from build123d import *

# Parameters (mm, degrees)
SKETCH_2_W          = 210
SKETCH_2_H          = 67
SKETCH_2_W_2        = 50
SKETCH_2_H_2        = 63
EXTRUDE_1_DEPTH     = 143
SKETCH_3_W          = 210
SKETCH_3_H          = 67
EXTRUDE_2_DEPTH     = 2
CUT_EXTRUDE_1_DEPTH = 5
SKETCH_5_W          = 210
SKETCH_5_H          = 145
CUT_EXTRUDE_2_DEPTH = 3
SKETCH_6_R          = 3.5
EXTRUDE_3_DEPTH     = 5
SKETCH_7_W          = 39
SKETCH_7_H          = 22
EXTRUDE_4_DEPTH     = 47
SKETCH_8_R          = 2.75
EXTRUDE_5_DEPTH     = 15
CUT_EXTRUDE_3_DEPTH = 288.697758073
FILLET_1_R          = 10
FILLET_2_R          = 4
EXTRUDE_6_DEPTH     = 5
FILLET_3_R          = 5
FILLET_4_R          = 2
SKETCH_11_W         = 210
SKETCH_11_H         = 49
CUT_EXTRUDE_4_DEPTH = 5
FILLET_5_R          = 5


# Some blends are built 0.0001 mm under size
with BuildPart() as part:
    # Эскиз2 → Бобышка-Вытянуть1 (new body)
    with BuildSketch(Plane.XY):
        with Locations((100, 28.5)):
            Rectangle(SKETCH_2_W, SKETCH_2_H)
        with Locations((22, 28.5)):
            Rectangle(SKETCH_2_W_2, SKETCH_2_H_2, mode=Mode.SUBTRACT)
        with Locations((74, 28.5)):
            Rectangle(SKETCH_2_W_2, SKETCH_2_H_2, mode=Mode.SUBTRACT)
        with Locations((126, 28.5)):
            Rectangle(SKETCH_2_W_2, SKETCH_2_H_2, mode=Mode.SUBTRACT)
        with Locations((178, 28.5)):
            Rectangle(SKETCH_2_W_2, SKETCH_2_H_2, mode=Mode.SUBTRACT)
    extrude(amount=EXTRUDE_1_DEPTH)

    # Эскиз3 → Бобышка-Вытянуть2 (add)
    with BuildSketch(Plane.XY.offset(143)):
        with Locations((100, 28.5)):
            Rectangle(SKETCH_3_W, SKETCH_3_H)
    extrude(amount=EXTRUDE_2_DEPTH)

    # Эскиз4 → Вырез-Вытянуть1 (cut)
    with BuildSketch(Plane.XZ.offset(5)):
        with BuildLine():
            Line((85.828427125, 143), (114.171572875, 143))
            ThreePointArc((114.171572875, 143), (115.319623172, 143.228361402), (116.292893219, 143.878679656))
            Line((116.292893219, 143.878679656), (118.414213562, 146))
            Line((118.414213562, 146), (81.585786438, 146))
            Line((81.585786438, 146), (83.707106781, 143.878679656))
            ThreePointArc((83.707106781, 143.878679656), (84.680376828, 143.228361402), (85.828427125, 143))
        make_face()
    extrude(amount=-CUT_EXTRUDE_1_DEPTH, mode=Mode.SUBTRACT)

    # Эскиз5 → Вырез-Вытянуть2 (cut)
    with BuildSketch(Plane(origin=(0, 62, 0), x_dir=(1, 0, 0), z_dir=(0, 1, 0))):
        with Locations((100, -72.5)):
            Rectangle(SKETCH_5_W, SKETCH_5_H)
    extrude(amount=-CUT_EXTRUDE_2_DEPTH, mode=Mode.SUBTRACT)

    # Эскиз6 → Бобышка-Вытянуть3 (add)
    # profile 1 of 4: a face of its own
    with BuildSketch(Plane.XZ.offset(5)):
        with BuildLine():
            Line((205, 22), (205, 39))
            Line((205, 39), (209, 39))
            ThreePointArc((209, 39), (217.5, 30.5), (209, 22))
            Line((209, 22), (205, 22))
        make_face()
        with Locations(Location((209, 30.5, 0), (0, 0, 270))):
            Circle(SKETCH_6_R, mode=Mode.SUBTRACT)
    # profile 2 of 4: a face of its own
    with BuildSketch(Plane.XZ.offset(5)):
        with BuildLine():
            Line((209, 47), (205, 47))
            Line((205, 47), (205, 64))
            Line((205, 64), (209, 64))
            ThreePointArc((209, 64), (217.5, 55.5), (209, 47))
        make_face()
        with Locations(Location((209, 55.5, 0), (0, 0, 270))):
            Circle(SKETCH_6_R, mode=Mode.SUBTRACT)
    # profile 3 of 4: a face of its own
    with BuildSketch(Plane.XZ.offset(5)):
        with BuildLine():
            Line((-5, 47), (-5, 64))
            Line((-5, 64), (-9, 64))
            ThreePointArc((-9, 64), (-17.5, 55.5), (-9, 47))
            Line((-9, 47), (-5, 47))
        make_face()
        with Locations(Location((-9, 55.5, 0), (0, 0, 90))):
            Circle(SKETCH_6_R, mode=Mode.SUBTRACT)
    # profile 4 of 4: a face of its own
    with BuildSketch(Plane.XZ.offset(5)):
        with BuildLine():
            Line((-9, 39), (-5, 39))
            Line((-5, 39), (-5, 22))
            Line((-5, 22), (-9, 22))
            ThreePointArc((-9, 22), (-17.5, 30.5), (-9, 39))
        make_face()
        with Locations(Location((-9, 30.5, 0), (0, 0, 90))):
            Circle(SKETCH_6_R, mode=Mode.SUBTRACT)
    extrude(amount=-EXTRUDE_3_DEPTH)

    # Эскиз7 → Бобышка-Вытянуть4 (add)
    with BuildSketch(Plane.XZ.offset(5)):
        with Locations((224.5, 11)):
            Rectangle(SKETCH_7_W, SKETCH_7_H)
    extrude(amount=-EXTRUDE_4_DEPTH)

    # Эскиз8 → Бобышка-Вытянуть5 (add)
    with BuildSketch(Plane.XZ.offset(-42)):
        with BuildLine():
            Line((239, 23), (217, 23))
            ThreePointArc((217, 23), (213.464466094, 21.535533906), (212, 18))
            Line((212, 18), (212, -29.15))
            ThreePointArc((212, -29.15), (213.464466094, -32.685533906), (217, -34.15))
            Line((217, -34.15), (239, -34.15))
            ThreePointArc((239, -34.15), (242.535533906, -32.685533906), (244, -29.15))
            Line((244, -29.15), (244, 18))
            ThreePointArc((244, 18), (242.535533906, 21.535533906), (239, 23))
        make_face()
        with Locations(Location((238.75, -5.575, 0), (0, 0, 270))):
            Circle(SKETCH_8_R, mode=Mode.SUBTRACT)
        with Locations(Location((217.25, -5.575, 0), (0, 0, 270))):
            Circle(SKETCH_8_R, mode=Mode.SUBTRACT)
    extrude(amount=EXTRUDE_5_DEPTH)

    # Эскиз9 → Вырез-Вытянуть3 (cut, through all)
    with BuildSketch(Plane(origin=(0, 42, 0), x_dir=(1, 0, 0), z_dir=(0, 1, 0))):
        with BuildLine():
            Line((239, -23), (235.274216073, -23))
            Line((235.274216073, -23), (246.59675483, -31.709945179))
            Line((246.59675483, -31.709945179), (255.697113083, -21.551405734))
            Line((255.697113083, -21.551405734), (244, -13.403410553))
            Line((244, -13.403410553), (244, -18))
            ThreePointArc((244, -18), (242.535533906, -21.535533906), (239, -23))
        make_face()
    extrude(amount=-CUT_EXTRUDE_3_DEPTH, mode=Mode.SUBTRACT)

    # Скругление1
    # the kernel refuses this fillet: 10 mm, written as the material it adds along each edge
    with BuildSketch(Plane(origin=(212, 66.874685928, 0), x_dir=(0, 0, -1), z_dir=(0, -1, 0))) as fillet_1_piece_1_section:
        with BuildLine():
            CenterArc((9.949874371, -10), FILLET_1_R, 90, 84.260829523)
            Line((0, -9), (0, 0))
            Line((0, 0), (9.949874371, 0))
        make_face()
    fillet_1_piece_1 = extrude(amount=39.874685928, mode=Mode.PRIVATE)
    fillet_1_piece_1 = split(fillet_1_piece_1, bisect_by=Plane(origin=(205, 50.5, -0.134473646), z_dir=(-1, 0, 0)), keep=Keep.TOP, mode=Mode.PRIVATE)
    fillet_1_piece_1 = split(fillet_1_piece_1, bisect_by=Plane(origin=(204.014524412, 59, -0.134473646), z_dir=(0, -1, 0)), keep=Keep.TOP, mode=Mode.PRIVATE)
    add(fillet_1_piece_1)
    with BuildSketch(Plane(origin=(212, 42, 0), x_dir=(0, 0, -1), z_dir=(0, -1, 0))) as fillet_1_piece_2:
        with BuildLine():
            CenterArc((9.949874371, -10), FILLET_1_R, 90, 84.260829523)
            Line((0, -9), (0, 0))
            Line((0, 0), (9.949874371, 0))
        make_face()
    extrude(amount=15)

    # Скругление2
    fillet_2_edges = [part.edges().sort_by_distance(p)[0] for p in [
        (209, -2.5, 22),
        (205, -2.5, 64),
        (205, -2.5, 47),
        (205, -2.5, 39),
    ]]
    fillet(fillet_2_edges, radius=FILLET_2_R - 0.0001)  # a hair under: the kernel refuses the full size

    # Эскиз10 → Бобышка-Вытянуть6 (add)
    with BuildSketch(Plane(origin=(0, 0, 0), x_dir=(1, 0, 0), z_dir=(0, 1, 0))):
        Polygon((217.5, -30.5), (217.5, -55.5), (206.060928994, -47), (205, -45.939071006), (205, -34.579189919), (213.295374463, -34.579189919), align=None)
    extrude(amount=-EXTRUDE_6_DEPTH)

    # Зеркальное отражение1: part across plane


with BuildPart() as part_1:
    add(part.part)
    add(part.part.mirror(Plane(origin=(100, 0, 0), x_dir=(0, 0, 1), z_dir=(1, 0, 0))))

    # Скругление3
    fillet_3_edges = [part_1.edges().sort_by_distance(p)[0] for p in [
        (205, 42, 10.794758822),
        (-5, 42, 10.794758822),
    ]]
    fillet(fillet_3_edges, radius=FILLET_3_R)

    # Скругление4
    fillet_4_edges = [part_1.edges().sort_by_distance(p)[0] for p in [
        (203, -3, 71.5),
        (178, -3, 143),
        (153, -3, 71.5),
        (203, 28, 143),
        (153, 28, 143),
        (151, 28, 143),
        (151, -3, 71.5),
        (101, -3, 71.5),
        (101, 29.5, 143),
        (99, 29.5, 143),
        (49, 28, 143),
        (-3, 28, 143),
        (-3, -3, 71.5),
        (47, 28, 143),
        (22, -3, 143),
        (47, -3, 71.5),
        (49, -3, 71.5),
        (99, -3, 71.5),
    ]]
    fillet(fillet_4_edges, radius=FILLET_4_R)

    # Эскиз11 → Вырез-Вытянуть4 (cut)
    with BuildSketch(Plane(origin=(0, 59, 0), x_dir=(1, 0, 0), z_dir=(0, 1, 0))):
        with Locations((100, -120.5)):
            Rectangle(SKETCH_11_W, SKETCH_11_H)
    extrude(amount=-CUT_EXTRUDE_4_DEPTH, mode=Mode.SUBTRACT)

    # Скругление5
    # the kernel refuses this fillet: 5 mm, written as the material it takes off along each edge
    with BuildSketch(Plane(origin=(165.5, 59, 96), x_dir=(0, -1, 0), z_dir=(-1, 0, 0)), Plane(origin=(113.5, 59, 96), x_dir=(0, -1, 0), z_dir=(-1, 0, 0)), Plane(origin=(61.5, 59, 96), x_dir=(0, -1, 0), z_dir=(-1, 0, 0)), Plane(origin=(217.5, 59, 96), x_dir=(0, -1, 0), z_dir=(-1, 0, 0))) as fillet_5_piece_1:
        with BuildLine():
            CenterArc((FILLET_5_R, -FILLET_5_R), FILLET_5_R, 90, 90)
            Line((0, -FILLET_5_R), (0, 0))
            Line((0, 0), (FILLET_5_R, 0))
        make_face()
    extrude(amount=27, mode=Mode.SUBTRACT)
    with BuildSketch(Plane(origin=(9.5, 59, 96), x_dir=(0, 0, -1), z_dir=(-1, 0, 0))) as fillet_5_piece_2:
        with BuildLine():
            CenterArc((FILLET_5_R, FILLET_5_R), FILLET_5_R, 180, 90)
            Line((0, FILLET_5_R), (0, 0))
            Line((0, 0), (FILLET_5_R, 0))
        make_face()
    extrude(amount=27, mode=Mode.SUBTRACT)


solid = part_1.part
CAD build for the part. Positions are in the model's coordinates, mm. A direction names the side the tool comes from. Round coordinates to 2 decimals unless told otherwise and drop trailing zeros. Write each loop counter-clockwise with the first axis right and the second up, starting at its lowest first coordinate (ties: lowest second). Pieces come first, ordered by that corner, then holes.
(1) Mould opens along X. For faces 4 (the face through (227, 42, -6)), 5 (the face through (178, -3, 70)), 6 (the face through (-14.94, -2.54, 61.58)), 7 (the face through (74, 26, 143)) say: pulls with the +X half, pulls with the -X half, needs draft (parallel to the pull), parting line crosses it, or undercut.
(2) Slice it at A-A, the plane x = 107.5. Write the cut outline in (y, z), and give its area (3 significant figures).
(3) Slice it at D-D, the plane x = 141. Write the cut outline in (y, z).
(4) Probe line 1 along X through (y, z) = (16, 86.5); line 2 along Z through (x, y) = (209, -1); line 3 along Z through (x, y) = (-38.75, 31) (3 decimals). List the from-to ranges inside material, lowest first.
(5) Slice it at C-C, the plane z = 75. Write the cut outline in (x, y), and give its area (3 significant figures).
(6) 3-axis set-ups, long thin cutter, end or side, ignore diameter. For faces 1 (the face through (214.94, -2.54, 61.58)), 2 (the face through (203, 29, 70)), 3 (the face through (100, 54, 131)): which of +Z, -Z, +X, -X, +Y, -Y reach the whole face in a straight line?
(7) Drop flat-ended pins along their axis: P1, Ø0.8, axis at x = 233.5, z = 22.5, coming from the -Y side; P2, Ø10, axis at x = 227, z = -15, coming from the +Y side; P3, Ø14, axis at x = 18.5, y = 28, coming from the -Z side. Give the stop position or say it passes through.
From the geometry:
1. face 4: needs draft
1. face 5: undercut
1. face 6: pulls with the -X half
1. face 7: undercut
2. outline: (-5, 0) - (-3, 0) - (-3, 143) - (-5, 143) - close; (0, 143) - (54, 143) - (54, 145) - (0, 145) - close
2. area: 394 mm2
3. outline: (-5, 0) - (-3, 0) - (-3, 143) - (54, 143) - (54, 145) - (-5, 145) - close
4. line 1: x = -5 to -3, 47 to 49, 99 to 101, 151 to 153, 203 to 205
4. line 2: z = 0 to 27, 34 to 52, 59 to 64
4. line 3: z = -34.15 to -8.325, -2.825 to 23
5. outline: (-5, -5) - (205, -5) - (205, 59) - (203, 59) - (203, -1) arc R2 cw to (201, -3) - (155, -3) arc R2 cw to (153, -1) - (153, 59) - (151, 59) - (151, -1) arc R2 cw to (149, -3) - (103, -3) arc R2 cw to (101, -1) - (101, 59) - (99, 59) - (99, -1) arc R2 cw to (97, -3) - (51, -3) arc R2 cw to (49, -1) - (49, 59) - (47, 59) - (47, -1) arc R2 cw to (45, -3) - (-1, -3) arc R2 cw to (-3, -1) - (-3, 59) - (-5, 59) - close
5. area: 1,050 mm2
6. face 1: +Z, +X, +Y, -Y
6. face 2: -Z, +Y
6. face 3: +Z, +X, -X, +Y
7. P1: stops at y = 27
7. P2: stops at y = 42
7. P3: stops at z = 143
